Could you check a few things on this model? Use its own coordinates, in mm. Give positions to 0.01 mm unless a question says otherwise; leave off trailing zeros. Loops run counter-clockwise (first coordinate to the right, second up) from the corner with the lowest first, then second, coordinate; pieces in that order, holes last. Notation, with made-up numbers: (-27.75, 24.5) - (19.25, 24.5) arc R22 ccw to (19.25, 61.5) - close; hole circle Ø6 at (-37.75, 53). An arc over 180 degrees is marked (long way). Use CSV: the item, a comma, the result in double quotes.
from build123d import *

# Parameters (mm, degrees)
SKETCH1_R               = 7.9375
SKETCH1_R_2             = 6.4643
BOSS_EXTRUDE1_DEPTH     = 295.474372219
CUT_EXTRUDE1_DEPTH      = 296.687525017
CUT_EXTRUDE1_DEPTH_BACK = 296.687525017


with BuildPart() as part:
    # Sketch1 → Boss-Extrude1 (new body)
    with BuildSketch(Plane(origin=(0, 0, 0), x_dir=(1, 0, 0), z_dir=(0, 1, 0))):
        with Locations(Location((0, 0, 0), (0, 0, 270))):
            Circle(SKETCH1_R)
        with Locations(Location((0, 0, 0), (0, 0, 270))):
            Circle(SKETCH1_R_2, mode=Mode.SUBTRACT)
    extrude(amount=BOSS_EXTRUDE1_DEPTH)

    # Sketch4 → Cut-Extrude1 (cut, two sides: drawn at the far end of the back side and taken through both)
    with BuildSketch(Plane(origin=(0, 0, 0), x_dir=(0, 0, -1), z_dir=(1, 0, 0)).offset(-CUT_EXTRUDE1_DEPTH_BACK)):
        with BuildLine():
            Line((3.175, 320.874372219), (3.175, 270.074372219))
            ThreePointArc((3.175, 270.074372219), (0, 266.899372219), (-3.175, 270.074372219))
            Line((-3.175, 270.074372219), (-3.175, 320.874372219))
            ThreePointArc((-3.175, 320.874372219), (0, 324.049372219), (3.175, 320.874372219))
        make_face()
    extrude(amount=CUT_EXTRUDE1_DEPTH + CUT_EXTRUDE1_DEPTH_BACK, mode=Mode.SUBTRACT)


solid = part.part
1) I need wall thicknesses on line 1 along Z through (x, y) = (0, 69); line 2 along Z through (x, y) = (-3.25, 80.5). Which ranges of each line are inside material? Lowest first, please.
Answer below:
line 1,"z = -7.94 to -6.46, 6.46 to 7.94"
line 2,"z = -7.24 to -5.59, 5.59 to 7.24"
2) Suppose I cut it at C-C (y = 123). Please give me the cut outline in (x, z) (1 decimal).
Answer below:
outline,"circle Ø15.9 at (0, 0); hole circle Ø12.9 at (0, 0)"
3) Suppose I cut it at B-B (x = 0). Please give me the cut outline in (y, z), plus the area to 3 significant figures.
Answer below:
outline,"(0, -7.94) - (295.47, -7.94) - (295.47, -6.46) - (0, -6.46) - close; (0, 6.46) - (295.47, 6.46) - (295.47, 7.94) - (0, 7.94) - close"
area,"871 mm2"
4) We'd pull the mould along Z, two halves only. Please class faces 1 (the flat face through (0, 295.474, 7)), 2 (the cylindrical face through (-3.04, 145.669, 7.332)), 3 (the cylindrical face through (6.41, 145.67, -0.84)): +Z half, -Z half, draft (parallel to the pull), parting line (faces both ways), or undercut.
Answer below:
face 1,"draft"
face 2,"parting line"
face 3,"undercut"
5) Suppose I cut it at A-A (z = 0). Please give me the cut outline in (x, y).
Answer below:
outline,"(-7.94, 0) - (-6.46, 0) - (-6.46, 266.9) - (-7.94, 266.9) - close; (6.46, 0) - (7.94, 0) - (7.94, 266.9) - (6.46, 266.9) - close"
6) I'm going to push flat-ended pins straight in: P1, Ø1, axis at y = 156, z = 2, coming from the +X side; P2, Ø5, axis at x = -5.5, y = 186.5, coming from the +Z side; P3, Ø5, axis at x = 6, y = 213.5, coming from the +Z side. Where does each tip first touch, or does it pass through?
Answer below:
P1,"stops at x = 7.79"
P2,"stops at z = 7.35"
P3,"stops at z = 7.12"
